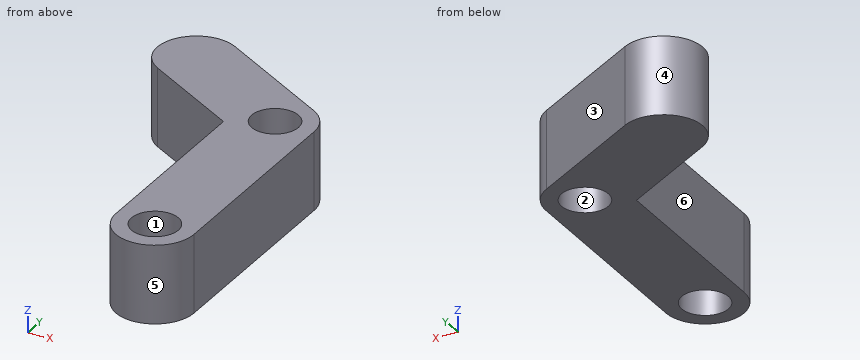
from build123d import *

# Parameters (mm, degrees)
SKIZZE1_R                       = 1.5
AUFSATZ_LINEAR_AUSTRAGEN1_DEPTH = 5


with BuildPart() as part:
    # Skizze1 → Aufsatz-Linear austragen1 (new body)
    with BuildSketch(Plane.XY):
        with BuildLine():
            ThreePointArc((-2.5, 0), (0, -2.5), (2.5, 0))
            Line((2.5, 0), (2.5, 13.78))
            ThreePointArc((2.5, 13.78), (2.170497036, 15.020541259), (1.268845907, 15.934072901))
            Line((1.268845907, 15.934072901), (-6.219211481, 20.344875789))
            ThreePointArc((-6.219211481, 20.344875789), (-9.64213029, 19.459648795), (-8.756903296, 16.036729986))
            Line((-8.756903296, 16.036729986), (-2.5, 12.351132282))
            Line((-2.5, 12.351132282), (-2.5, 0))
        make_face()
        Circle(SKIZZE1_R, mode=Mode.SUBTRACT)
        with Locations((0, 13.78)):
            Circle(SKIZZE1_R, mode=Mode.SUBTRACT)
    extrude(amount=AUFSATZ_LINEAR_AUSTRAGEN1_DEPTH)


solid = part.part
Verification items for the finished model (mm, model axes). Face numbers are marked on the shaded views. A direction names the side the tool comes from. Coordinates: 2 decimals unless noted, no trailing zeros. Order: outer loops, then holes, each group sorted by start corner. A loop starts at its lowest first (then second) coordinate and runs counter-clockwise, first axis right, second up. Notation, with made-up numbers: M 14,71 L 28,71 A27 cw 28,101 Z; hole C 24,-6.5 d5. An arc over 180 degrees is marked long. One line per item, written item: value. Start each with the question number.
Item 1: Access from +Z, -Z, +X, -X, +Y, -Y to the whole of each face (thin tool, end or side, straight path). Record for the marked faces 5 and 6.
Item 2: Depth check by flat-ended pin: P1, Ø3, axis at x = -1.5, z = 0.5, coming from the +Y side; P2, Ø1.5, axis at y = 17, z = 2, coming from the -X side; P3, Ø1.5, axis at y = 9, z = 2, coming from the -X side. Enter the tip coordinate at first touch or a pass-through.
Item 3: Thickness scan on probe 1 along Y at (x, z) = (0, 2.3); probe 2 along Y at (x, z) = (-0.5, 1.2); probe 3 along X at (y, z) = (12.5, 4.45). Record the ranges inside material, lowest first.
Item 4: Sectioned sample at D-D on y = 10.75. Record the cut outline in (x, z).
Item 5: Sectioned sample at A-A on z = 2.15. Record the cut outline in (x, y).
Item 6: Mould release check, pull along X, two halves, no side actions. Record for the marked faces 1, 2, 3 and 4: pulls with the +X half, pulls with the -X half, needs draft (parallel to the pull), parting line crosses it, or undercut.
Item 7: Sectioned sample at C-C on y = 13.25. Record the cut outline in (x, z).
Item 8: Sectioned sample at B-B on x = 0. Record the cut outline in (y, z).
Calculated:
1. face 5: +Z, -Z, -Y
1. face 6: +Z, -Z, -X, -Y
2. P1: y = 18.45
2. P2: x = -9.95
2. P3: x = -2.5
3. probe 1: -2.5 to -1.5, 1.5 to 12.28, 15.28 to 16.68
3. probe 2: -2.45 to -1.41, 1.41 to 12.37, 15.19 to 16.98
3. probe 3: -2.75 to -0.78, 0.78 to 2.5
4. outline: M -2.5,0 L 2.5,0 L 2.5,5 L -2.5,5 Z
5. outline: M -8.76,16.04 L -2.5,12.35 L -2.5,0 A2.5 ccw 2.5,0 L 2.5,13.78 A2.5 ccw 1.27,15.93 L -6.22,20.34 A2.5 ccw Z; hole C 0,0 d3; hole C 0,13.78 d3
6. face 1: undercut
6. face 2: undercut
6. face 3: pulls with the +X half
6. face 4: parting line crosses it
7. outline: M -4.03,0 L -1.4,0 L -1.4,5 L -4.03,5 Z; M 1.4,0 L 2.5,0 L 2.5,5 L 1.4,5 Z
8. outline: M -2.5,0 L -1.5,0 L -1.5,5 L -2.5,5 Z; M 1.5,0 L 12.28,0 L 12.28,5 L 1.5,5 Z; M 15.28,0 L 16.68,0 L 16.68,5 L 15.28,5 Z
